Design review of the part built by this model. Coordinates are the model's own, in mm. Coordinates: 2 decimals unless noted, no trailing zeros. Write each loop counter-clockwise with the first axis right and the second up, starting at its lowest first coordinate (ties: lowest second). Pieces come first, ordered by that corner, then holes.
Q1. Add section C-C, the plane z = 11.5. Give the boundary of the cut face in (x, y), plus the area to 3 significant figures.
Q2. Clearance check with flat-ended pins moving along their axes: pin 1 Ø6 at (y, z) = (-216.5, -26.5) entering from +X; pin 2 Ø6 at (x, z) = (158.5, -21.5) entering from +Y; pin 3 Ø8 at (y, z) = (73, 24) entering from +X. State where each tip first meets the part, or that it passes through.
Q3. Add section B-B, the plane z = -19.5. Give the boundary of the cut face in (x, y).
Q4. Add section A-A, the plane x = 0. Give the boundary of the cut face in (y, z), plus the area to 3 significant figures.
Q5. To check wall thickness, follow probe 1 along X at (y, z) = (-44, -3); probe 2 along Y at (x, z) = (0, 0); probe 3 along Z at (x, y) = (106, -235). State the ranges of each line that lie inside material, in increasing order.
from build123d import *

# Parameters (mm, degrees)
SKETCH1_R           = 250.932647595
BOSS_EXTRUDE1_DEPTH = 35
FILLET1_R           = 30
SKETCH2_R           = 175
CUT_EXTRUDE1_DEPTH  = 70


with BuildPart() as part:
    # Sketch1 → Boss-Extrude1 (new, symmetric)
    with BuildSketch(Plane.XY):
        with Locations((0, -38.296576895)):
            Circle(SKETCH1_R)
    extrude(amount=BOSS_EXTRUDE1_DEPTH, both=True)

    # Fillet1
    fillet1_edges = [part.edges().sort_by_distance(p)[0] for p in [
        (-250.932647595, -38.296576895, -35),
        (-250.932647595, -38.296576895, 35),
    ]]
    fillet(fillet1_edges, radius=FILLET1_R)

    # Sketch2 → Cut-Extrude1 (cut)
    with BuildSketch(Plane.XY.offset(35)):
        with Locations((0, -38.296576895)):
            Circle(SKETCH2_R)
    extrude(amount=-CUT_EXTRUDE1_DEPTH, mode=Mode.SUBTRACT)


solid = part.part
Here are the results:
1. outline: circle Ø500.44 at (0, -38.3); hole circle Ø350 at (0, -38.3)
1. area: 100,000 mm2
2. pin 1: stops at x = 168.69
2. pin 2: stops at y = 153.24
2. pin 3: stops at x = 221.07
3. outline: circle Ø494.39 at (0, -38.3); hole circle Ø350 at (0, -38.3)
4. outline: (-289.23, -5) arc R30 ccw to (-259.23, -35) - (-213.3, -35) - (-213.3, 35) - (-259.23, 35) arc R30 ccw to (-289.23, 5) - close; (136.7, -35) - (182.64, -35) arc R30 ccw to (212.64, -5) - (212.64, 5) arc R30 ccw to (182.64, 35) - (136.7, 35) - close
4. area: 9,860 mm2
5. probe 1: x = -250.87 to -174.91, 174.91 to 250.87
5. probe 2: y = -289.23 to -213.3, 136.7 to 212.64
5. probe 3: z = -34.89 to 34.89
